Here's how the part is built. I have some questions about the finished solid (model axes, mm). Coordinates: 2 decimals unless noted, no trailing zeros. Write each loop counter-clockwise with the first axis right and the second up, starting at its lowest first coordinate (ties: lowest second). Pieces come first, ordered by that corner, then holes.
(1) Imagine slicing it at C-C, the plane y = 1.1. List the corners of the cut face in (x, z) for me.
(2) Please list where these lines run through material, in increasing order: probe 1 along Z at (x, y) = (0, -0.1); probe 2 along Z at (x, y) = (0, 1.4); probe 3 along Y at (x, z) = (-4.75, 8.75).
(3) Imagine slicing it at D-D, the plane x = 6.5. List the corners of the cut face in (y, z) for me.
(4) Imagine slicing it at B-B, the plane z = 3.5. List the corners of the cut face in (x, y) for me.
(5) For pin 1 Ø1.2 at (x, z) = (0, 3.5) entering from +Y; pin 2 Ø2 at (x, z) = (-4, -6) entering from -Y, each with a flat end and sliding along its axis, tell me the tip position at first contact or that it passes through.
(6) Imagine slicing it at A-A, the plane x = 0. List the corners of the cut face in (y, z) for me, plus the area to 3 significant figures.
(7) Thinking about a two-plate mould opening in Z: for faces 1 (the cylindrical face through (-0.13, 0.99, 4.49)), 2 (the cylindrical face through (0.954, 0.986, -3.2)), 3 (the flat face through (0, 1, 10)), 4 (the flat face through (3, 0, 0)), which applies, released by +Z, released by -Z, zero draft, split by the parting line, or undercut?
Solid Edge part; units mm, degrees
sketch "Sketch1" plane through (0, 0, 0) normal (0, -1, 0) x (1, 0, 0)
  line L0 (7.5, 10) -> (-7.5, 10)
  line L1 (-7.5, 10) -> (-7.5, -10)
  line L2 (-7.5, -10) -> (7.5, -10)
  line L3 (7.5, -10) -> (7.5, 10)
  circle A0 centre (0, 3.5) radius 1
  circle A1 centre (0, -3.5) radius 1
extrude "Protrusion1" add sketch "Sketch1" against normal blind 2
sketch "Sketch2" plane through (0, 0, 0) normal (0, -1, 0) x (1, 0, 0)
  line L0 (2.5, -5) -> (2.5, 5)
  line L1 (2.5, 5) -> (-2.5, 5)
  line L2 (-2.5, 5) -> (-2.5, -5)
  line L3 (-2.5, -5) -> (2.5, -5)
  circle A0 centre (0, 3.5) radius 1.1
  circle A1 centre (0, -3.5) radius 1.1
extrude "ExtrudedProtrusion_2" add sketch "Sketch2" along normal blind 0.25
Recorded:
1. outline: (-7.5, -10) - (7.5, -10) - (7.5, 10) - (-7.5, 10) - close; hole circle Ø2 at (0, -3.5); hole circle Ø2 at (0, 3.5)
2. probe 1: z = -5 to -4.6, -2.4 to 2.4, 4.6 to 5
2. probe 2: z = -10 to -4.5, -2.5 to 2.5, 4.5 to 10
2. probe 3: y = 0 to 2
3. outline: (0, -10) - (2, -10) - (2, 10) - (0, 10) - close
4. outline: (-7.5, 0) - (-2.5, 0) - (-2.5, -0.25) - (-1.1, -0.25) - (-1.1, 0) - (-1, 0) - (-1, 2) - (-7.5, 2) - close; (1, 0) - (1.1, 0) - (1.1, -0.25) - (2.5, -0.25) - (2.5, 0) - (7.5, 0) - (7.5, 2) - (1, 2) - close
5. pin 1: passes through
5. pin 2: stops at y = 0
6. outline: (-0.25, -5) - (0, -5) - (0, -10) - (2, -10) - (2, -4.5) - (0, -4.5) - (0, -4.6) - (-0.25, -4.6) - close; (-0.25, -2.4) - (0, -2.4) - (0, -2.5) - (2, -2.5) - (2, 2.5) - (0, 2.5) - (0, 2.4) - (-0.25, 2.4) - close; (-0.25, 4.6) - (0, 4.6) - (0, 4.5) - (2, 4.5) - (2, 10) - (0, 10) - (0, 5) - (-0.25, 5) - close
6. area: 33.4 mm2
7. face 1: undercut
7. face 2: undercut
7. face 3: released by +Z
7. face 4: zero draft
